Verification items for the finished model (mm, model axes). Face numbers are marked on the shaded views. A direction names the side the tool comes from. Give positions to 0.01 mm unless a question says otherwise; leave off trailing zeros. Loops run counter-clockwise (first coordinate to the right, second up) from the corner with the lowest first, then second, coordinate; pieces in that order, holes last. Notation, with made-up numbers: (75, 47) -> (86, 47) arc R36 ccw to (86, 84) -> close; hole circle Ø9 at (85, 58). An arc over 180 degrees is marked (long way). Answer in a Markdown table with one row per item. Add a question column.
Q1. Section check D-D on y = 3.5. Enter the section's corners in (x, z).
Q2. Gauge pin test, flat ends, axial feed: P1, Ø5, axis at x = 1, y = -0.5, coming from the -Z side; P2, Ø1.3, axis at y = -0.5, z = -4, coming from the -X side; P3, Ø3, axis at y = -1.5, z = -5.5, coming from the +X side; P4, Ø8, axis at x = -4.5, y = 4.5, coming from the +Z side. Record the tip position at first contact, or that the pin passes through.
Q3. Set-up check for the marked faces 4, 5 and 6: record each of +Z, -Z, +X, -X, +Y, -Y from which the full face is reachable in a straight line by a thin tool's end or side.
Q4. Release check for a two-part mould opening along X. For the marked faces 1, 2 and 3 record: pulls with the +X half, pulls with the -X half, needs draft (parallel to the pull), parting line crosses it, or undercut.
Q5. Section check A-A on y = 0. Enter the section's corners in (x, z).
Q6. Section check B-B on z = -2.5. Enter the section's corners in (x, y).
Q7. Material ranges on probe 1 along Z at (x, y) = (8.25, 1); probe 2 along Z at (x, y) = (11, -2.25); probe 3 along X at (y, z) = (-2, -0.5), recorded low to high.
Q8. Section check C-C on x = 4. Enter the section's corners in (y, z).
```python
from build123d import *

# Parameters (mm, degrees)
PAD005_DEPTH = 10
SKETCH014_R  = 1.5
PAD013_DEPTH = 10
SKETCH002_R  = 6
PAD001_DEPTH = 2.6
SKETCH003_R  = 2.6
PAD002_DEPTH = 7.1
SKETCH004_R  = 4.5
PAD003_DEPTH = 10
SKETCH005_R  = 6.5
PAD004_DEPTH = 4.2
PAD006_DEPTH = 2


with BuildPart() as motor_linkage_hole_body:
    # Sketch006 → Pad005 (new body)
    with BuildSketch(Plane.XY):
        with BuildLine():
            Line((-7, 2.236068), (-7, -2.236068))
            ThreePointArc((-7, -2.236068), (-5, -3), (-3, -2.236068))
            Line((-3, -2.236068), (-3, 2.236068))
            ThreePointArc((-3, 2.236068), (-5, 3), (-7, 2.236068))
        make_face()
    extrude(amount=-PAD005_DEPTH)


with BuildPart() as hole_fusion:
    # Sketch014 → Pad013 (new body, symmetric)
    with BuildSketch(Plane.XY):
        with Locations((5.020646, 0)):
            Circle(SKETCH014_R)
    extrude(amount=PAD013_DEPTH, both=True)

    # Fusion005: union motor linkage hole body
    add(motor_linkage_hole_body.part)


with BuildPart() as motor_linkage_cut:
    # Sketch002 → Pad001 (new body)
    with BuildSketch(Plane.XY):
        with Locations((5, 0)):
            Circle(SKETCH002_R)
    extrude(amount=PAD001_DEPTH)

    # Sketch003 → Pad002 (join)
    with BuildSketch(Plane.XY):
        with Locations((5, 0)):
            Circle(SKETCH003_R)
    extrude(amount=PAD002_DEPTH)

    # Sketch004 → Pad003 (join)
    with BuildSketch(Plane.XY):
        with Locations((-5, 0)):
            Circle(SKETCH004_R)
    extrude(amount=-PAD003_DEPTH)

    # Sketch005 → Pad004 (join)
    with BuildSketch(Plane.XY):
        with Locations((-5, 0)):
            Circle(SKETCH005_R)
    extrude(amount=-PAD004_DEPTH)

    # Sketch001 → Pad006 (join)
    with BuildSketch(Plane.XY):
        with BuildLine():
            Line((-5, 8), (5, 8))
            ThreePointArc((5, -8), (13, 0), (5, 8))
            Line((-5, -8), (5, -8))
            ThreePointArc((-5, 8), (-13, 0), (-5, -8))
        make_face()
    extrude(amount=PAD006_DEPTH)

    # Cut: cut hole fusion
    add(hole_fusion.part, mode=Mode.SUBTRACT)


solid = motor_linkage_cut.part
```
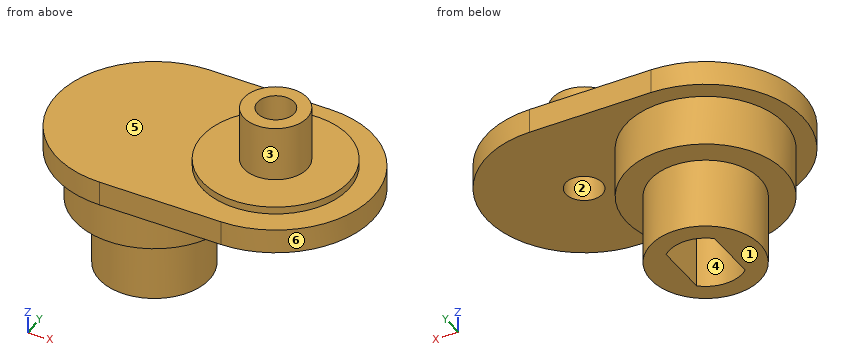
Taken from the geometry:
| question | item | result |
|---|---|---|
| 1 | outline | (-12.19, 0) -> (-10.48, 0) -> (-10.48, -4.2) -> (-7.83, -4.2) -> (-7.83, -10) -> (-2.17, -10) -> (-2.17, -4.2) -> (0.48, -4.2) -> (0.48, 0) -> (12.19, 0) -> (12.19, 2) -> (9.87, 2) -> (9.87, 2.6) -> (0.13, 2.6) -> (0.13, 2) -> (-12.19, 2) -> close |
| 2 | P1 | stops at z = -10 |
| 2 | P2 | stops at x = -11.5 |
| 2 | P3 | stops at x = 1.46 |
| 2 | P4 | stops at z = 2 |
| 3 | face 4 | -Z |
| 3 | face 5 | +Z |
| 3 | face 6 | +Z, -Z, +X |
| 4 | face 1 | needs draft |
| 4 | face 2 | undercut |
| 4 | face 3 | parting line crosses it |
| 5 | outline | (-13, 0) -> (-11.5, 0) -> (-11.5, -4.2) -> (-9.5, -4.2) -> (-9.5, -10) -> (-7, -10) -> (-7, 0) -> (-3, 0) -> (-3, -10) -> (-0.5, -10) -> (-0.5, -4.2) -> (1.5, -4.2) -> (1.5, 0) -> (3.52, 0) -> (3.52, 7.1) -> (2.4, 7.1) -> (2.4, 2.6) -> (-1, 2.6) -> (-1, 2) -> (-13, 2) -> close; (6.52, 0) -> (13, 0) -> (13, 2) -> (11, 2) -> (11, 2.6) -> (7.6, 2.6) -> (7.6, 7.1) -> (6.52, 7.1) -> close |
| 6 | outline | circle Ø13 at (-5, 0); hole (-7, -2.24) arc R3 ccw to (-3, -2.24) -> (-3, 2.24) arc R3 ccw to (-7, 2.24) -> close |
| 7 | probe 1 | z = 0 to 2.6 |
| 7 | probe 2 | z = 0 to 2 |
| 7 | probe 3 | x = -11.18 to -7, -3 to 1.18 |
| 8 | outline | (-8, 0) -> (-1.1, 0) -> (-1.1, 7.1) -> (-2.4, 7.1) -> (-2.4, 2.6) -> (-5.92, 2.6) -> (-5.92, 2) -> (-8, 2) -> close; (1.1, 0) -> (8, 0) -> (8, 2) -> (5.92, 2) -> (5.92, 2.6) -> (2.4, 2.6) -> (2.4, 7.1) -> (1.1, 7.1) -> close |
